Answer from the drawing. Dimensions are ordinates in mm from the lowest x, y and z of the part. Coordinates: 2 decimals unless noted, no trailing zeros. Order: outer loops, then holes, each group sorted by start corner. A loop starts at its lowest first (then second) coordinate and runs counter-clockwise, first axis right, second up. Notation, with made-up numbers: (53.25, -9.5) -> (75.25, -9.5) arc R26 ccw to (75.25, 17.5) -> close; hole circle Ø6 at (68, 32.25). An arc over 180 degrees is marked (long way). Answer in a Markdown table with one row per item.
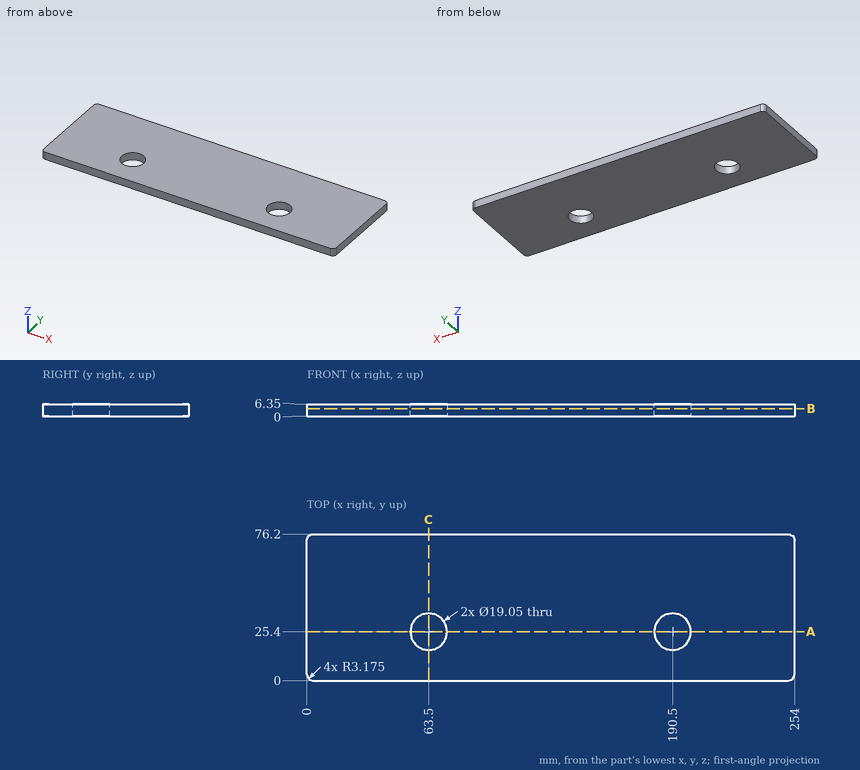
Q1. The part is cut by section B-B (z = 4). Write down the section's boundary in (x, y) (3 decimals).
Outcome:
| item | result |
|---|---|
| outline | (0, 3.175) arc R3.175 ccw to (3.175, 0) -> (250.825, 0) arc R3.175 ccw to (254, 3.175) -> (254, 73.025) arc R3.175 ccw to (250.825, 76.2) -> (3.175, 76.2) arc R3.175 ccw to (0, 73.025) -> close; hole circle Ø19.05 at (63.5, 25.4); hole circle Ø19.05 at (190.5, 25.4) |
Q2. Consider line 1 (Y direction, x = 63, z = 1.75); line 2 (X direction, y = 20, z = 5.75); line 3 (X direction, y = 33.5, z = 1.5). Determine where each line is inside the solid, lowest interval first.
Outcome:
| item | result |
|---|---|
| line 1 | 0 to 15.89, 34.91 to 76.2 |
| line 2 | 0 to 55.65, 71.35 to 182.65, 198.35 to 254 |
| line 3 | 0 to 58.49, 68.51 to 185.49, 195.51 to 254 |
Q3. Given pin 1 (15 mm diameter, centred on x = 190.5, y = 25.4, fed in from -Z), flat-ended and moving along its own axis, determine where the tip first touches the part or whether it passes through.
Outcome:
| item | result |
|---|---|
| pin 1 | through |
Q4. The part is cut by section C-C (x = 63.5). Write down the section's boundary in (y, z) (3 decimals), then the cut area to 3 significant figures.
Outcome:
| item | result |
|---|---|
| outline | (0, 0) -> (15.875, 0) -> (15.875, 6.35) -> (0, 6.35) -> close; (34.925, 0) -> (76.2, 0) -> (76.2, 6.35) -> (34.925, 6.35) -> close |
| area | 363 mm² |
Q5. The part is cut by section A-A (y = 25.4). Write down the section's boundary in (x, z) (3 decimals).
Outcome:
| item | result |
|---|---|
| outline | (0, 0) -> (53.975, 0) -> (53.975, 6.35) -> (0, 6.35) -> close; (73.025, 0) -> (180.975, 0) -> (180.975, 6.35) -> (73.025, 6.35) -> close; (200.025, 0) -> (254, 0) -> (254, 6.35) -> (200.025, 6.35) -> close |
